Geometry check sheet. Reference: the model listing, model coordinates, mm. A direction names the side the tool comes from. Coordinates: 2 decimals unless noted, no trailing zeros. Write each loop counter-clockwise with the first axis right and the second up, starting at its lowest first coordinate (ties: lowest second). Pieces come first, ordered by that corner, then holes. Notation, with made-up numbers: M -23.75,-8 L -13.75,-8 A29 ccw -13.75,28 Z; hole C -35,51 d5. An arc over 180 degrees is marked long. Put each result on its own line as item: value. Start each with the question number.
1) Gauge pin test, flat ends, axial feed: pin 1 (3 mm diameter, centred on y = 0.5, z = -3.5, fed in from +X); pin 2 (7.5 mm diameter, centred on x = 1.5, z = -1.5, fed in from +Y); pin 3 (1 mm diameter, centred on y = 1.5, z = 1, fed in from +X). Record the tip position at first contact, or that the pin passes through.
2) Cross-section at B-B on z = 0. Record the cut outline in (x, y).
3) Cross-section at C-C on y = 0.5. Record the cut outline in (x, z).
4) Set-up check for faces 5 (the flat face through (0, 2.4, -5)), 6 (the flat face through (0, 2.5, -8)): record each of +Z, -Z, +X, -X, +Y, -Y from which the full face is reachable in a straight line by a thin tool's end or side.
5) Scan lines: line 1 along Z through (x, y) = (0, -0.6); line 2 along Y through (x, z) = (-3, 4.5); line 3 along Z through (x, y) = (4, -1.9). Record each from-to range of solid material in increasing order.
6) Mould release check, pull along Z, two halves, no side actions. Record for faces 1 (the flat face through (0, -2.4, -5)), 2 (the flat face through (0, -2.5, -8)), 3 (the cylindrical face through (-3.233, -0.035, 1.341)), 4 (the cylindrical face through (-4.57, -0.035, -7.167)): released by +Z, released by -Z, zero draft, split by the parting line, or undercut.
7) Cross-section at A-A on x = 0. Record the cut outline in (y, z).
8) Cross-section at D-D on z = -4.25. Record the cut outline in (x, y), plus the area to 3 significant figures.
Autodesk Inventor part; units mm, degrees
ref_plane "YZ Plane" through (0, 0, 0) normal (1, 0, 0) x (0, 1, 0)
ref_plane "XZ Plane" through (0, 0, 0) normal (0, 1, 0) x (-1, 0, 0)
ref_plane "XY Plane" through (0, 0, 0) normal (0, 0, 1) x (1, 0, 0)
sketch "Skizze1" plane through (0, 0, 0) normal (0, 1, 0) x (-1, 0, 0)
  circle A0 centre (0, 0) radius 8.5
  circle A1 centre (0, 0) radius 3.5
  circle A2 centre (0, 0) radius 7.5
  circle A3 centre (0, 0) radius 4.5
  dimension "d0" = 17
  dimension "d1" = 7
  dimension "d2" = 1
  dimension "d3" = 1
extrude "Extrusion1" add sketch "Skizze1" along normal mid plane 5
extrude "Extrusion2" add sketch "Skizze1" along normal mid plane 4.8 contours A2
properties part number "Kugellager 14 x 7 x 5"
Answer key:
1. pin 1: stops at x = 8.26
1. pin 2: stops at y = 2.5
1. pin 3: stops at x = 8.49
2. outline: M -8.5,-2.5 L -7.5,-2.5 L -7.5,-2.4 L -4.5,-2.4 L -4.5,-2.5 L -3.5,-2.5 L -3.5,2.5 L -4.5,2.5 L -4.5,2.4 L -7.5,2.4 L -7.5,2.5 L -8.5,2.5 Z; M 3.5,-2.5 L 4.5,-2.5 L 4.5,-2.4 L 7.5,-2.4 L 7.5,-2.5 L 8.5,-2.5 L 8.5,2.5 L 7.5,2.5 L 7.5,2.4 L 4.5,2.4 L 4.5,2.5 L 3.5,2.5 Z
3. outline: C 0,0 d17; hole C 0,0 d7
4. face 5: +Y
4. face 6: +Z, -Z, +X, -X, +Y
5. line 1: z = -8.5 to -3.5, 3.5 to 8.5
5. line 2: y = -2.4 to 2.4
5. line 3: z = -7.5 to 7.5
6. face 1: undercut
6. face 2: zero draft
6. face 3: undercut
6. face 4: split by the parting line
7. outline: M -2.5,-8.5 L 2.5,-8.5 L 2.5,-7.5 L 2.4,-7.5 L 2.4,-4.5 L 2.5,-4.5 L 2.5,-3.5 L -2.5,-3.5 L -2.5,-4.5 L -2.4,-4.5 L -2.4,-7.5 L -2.5,-7.5 Z; M -2.5,3.5 L 2.5,3.5 L 2.5,4.5 L 2.4,4.5 L 2.4,7.5 L 2.5,7.5 L 2.5,8.5 L -2.5,8.5 L -2.5,7.5 L -2.4,7.5 L -2.4,4.5 L -2.5,4.5 Z
8. outline: M -7.36,-2.5 L -6.18,-2.5 L -6.18,-2.4 L -1.48,-2.4 L -1.48,-2.5 L 1.48,-2.5 L 1.48,-2.4 L 6.18,-2.4 L 6.18,-2.5 L 7.36,-2.5 L 7.36,2.5 L 6.18,2.5 L 6.18,2.4 L 1.48,2.4 L 1.48,2.5 L -1.48,2.5 L -1.48,2.4 L -6.18,2.4 L -6.18,2.5 L -7.36,2.5 Z
8. area: 71.7 mm²
